Job drawing, mm, ordinate dimensions from the low corner. One solid piece. A direction names the side the tool comes from. Give positions to 0.01 mm unless a question says otherwise; leave off trailing zeros. Order: outer loops, then holes, each group sorted by start corner. A loop starts at its lowest first (then second) coordinate and runs counter-clockwise, first axis right, second up. Notation, with made-up numbers: (27.5, -29.75) - (73.5, -29.75) arc R24 cw to (73.5, 5.25) - close; hole circle Ø11 at (-8, 68.25). An arc over 180 degrees is marked (long way). Write each question's results on one line, items separated by ' | '. Start each with the question number.
1) Cut at B-B on z = 63.5. List the corners of the cut face in (x, y).
2) Two-plate mould, pull along Y, no slides. Class the marked faces 1, 2 and 3: +Y half, -Y half, draft (parallel to the pull), parting line (faces both ways), or undercut.
3) Drop flat-ended pins along their axis: pin 1 Ø4 at (y, z) = (41, 98.5) entering from +X; pin 2 Ø6.5 at (y, z) = (102.616, 63.5) entering from -X; pin 3 Ø3 at (x, y) = (3.5, 38) entering from -Z; pin 4 Ø5 at (x, z) = (3, 98.5) entering from +Y. Give the stop position or say it passes through.
4) Cut at A-A on y = 63.5. List the corners of the cut face in (x, z).
5) Tool access for the marked faces 4 and 5: list every direction of +Z, -Z, +X, -X, +Y, -Y with a clear straight run to the whole face (end or side of a thin tool).
6) Cut at D-D on x = 9. State how many separate pieces and enclosed holes the cut face has, plus the area to 3 significant figures.
7) Drill centre lines: line 1 along Y through (x, z) = (10.5, 63.5); line 2 along Y through (x, z) = (1.05, 63.5); line 3 along X through (y, z) = (44.5, 8). Where is each one in solid material? Low to high. Write a range as from..to.
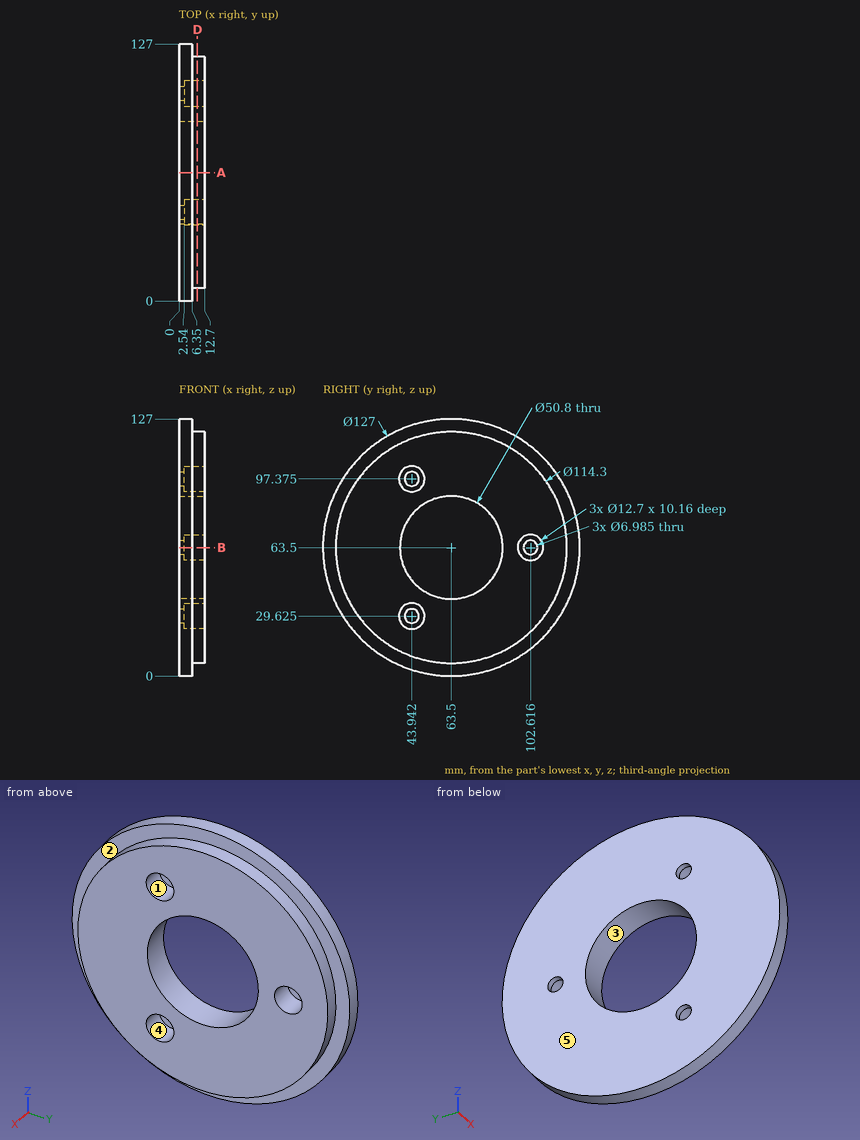
Results:
1) outline: (0, 0) - (6.35, 0) - (6.35, 6.35) - (12.7, 6.35) - (12.7, 38.1) - (0, 38.1) - close; (0, 88.9) - (12.7, 88.9) - (12.7, 96.27) - (2.54, 96.27) - (2.54, 99.12) - (0, 99.12) - close; (0, 106.11) - (2.54, 106.11) - (2.54, 108.97) - (12.7, 108.97) - (12.7, 120.65) - (6.35, 120.65) - (6.35, 127) - (0, 127) - close
2) face 1: undercut | face 2: draft | face 3: undercut
3) pin 1: x = 2.54 | pin 2: through | pin 3: z = 4.71 | pin 4: y = 118.05
4) outline: (0, 0) - (6.35, 0) - (6.35, 6.35) - (12.7, 6.35) - (12.7, 38.1) - (0, 38.1) - close; (0, 88.9) - (12.7, 88.9) - (12.7, 120.65) - (6.35, 120.65) - (6.35, 127) - (0, 127) - close
5) face 4: +X | face 5: +Z, -Z, -X, +Y, -Y
6) separate pieces: 1 | enclosed holes: 4 | area: 7,850 mm^2
7) line 1: 6.35..38.1, 88.9..96.27, 108.97..120.65 | line 2: 0..38.1, 88.9..99.12, 106.11..127 | line 3: 0..6.35
